Here's the drawing with two shaded views (mm, measured from the low corner). I have some questions. Round coordinates to 2 decimals unless told otherwise and drop trailing zeros. Order: outer loops, then holes, each group sorted by start corner. A loop starts at its lowest first (then second) coordinate and runs counter-clockwise, first axis right, second up. Notation, with made-up numbers: (-32.5, 65.25) -> (23.5, 65.25) arc R16 cw to (23.5, 87.25) -> close; hole circle Ø1 at (78, 86.25). An arc over 180 degrees is marked (long way). One line per question, with ' | ' between items.
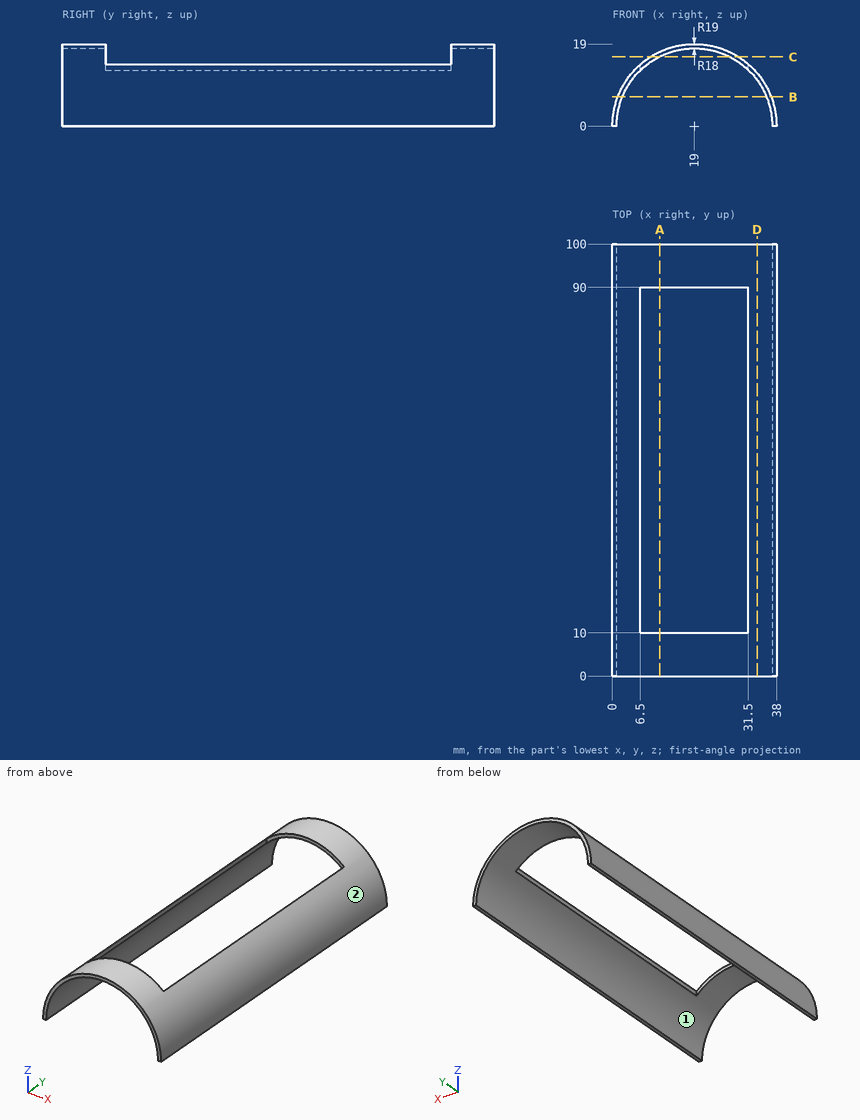
1. I want a section at C-C on z = 16. List the corners of the cut face in (x, y) for me.
From the geometry:
outline: (8.75, 0) -> (10.75, 0) -> (10.75, 10) -> (8.75, 10) -> close; (8.75, 90) -> (10.75, 90) -> (10.75, 100) -> (8.75, 100) -> close; (27.25, 0) -> (29.25, 0) -> (29.25, 10) -> (27.25, 10) -> close; (27.25, 90) -> (29.25, 90) -> (29.25, 100) -> (27.25, 100) -> close
2. I want a section at A-A on x = 11. List the corners of the cut face in (y, z) for me.
From the geometry:
outline: (0, 16.12) -> (10, 16.12) -> (10, 17.23) -> (0, 17.23) -> close; (90, 16.12) -> (100, 16.12) -> (100, 17.23) -> (90, 17.23) -> close
3. If we mould it in two halves opening along X, with no side actions, what happens to the marked faces 1 and 2? For each: pulls with the +X half, pulls with the -X half, needs draft (parallel to the pull), parting line crosses it, or undercut.
From the geometry:
face 1: undercut | face 2: parting line crosses it
4. I want a section at B-B on z = 6.75. List the corners of the cut face in (x, y) for me, and give its area (3 significant figures).
From the geometry:
outline: (1.24, 0) -> (2.31, 0) -> (2.31, 100) -> (1.24, 100) -> close; (35.69, 0) -> (36.76, 0) -> (36.76, 100) -> (35.69, 100) -> close | area: 215 mm²
5. I'm going to push flat-ended pins straight in: pin 1 (3 mm diameter, centred on x = 21.5, z = 15.5, fed in from +Y); pin 2 (1 mm diameter, centred on y = 11, z = 10.5, fed in from -X); pin 3 (1.5 mm diameter, centred on x = 4, y = 23, fed in from +Z); pin 4 (3 mm diameter, centred on x = 14.5, z = 17, fed in from -Y). Where does each tip first touch, or does it pass through?
From the geometry:
pin 1: passes through | pin 2: stops at x = 2.84 | pin 3: stops at z = 12.57 | pin 4: stops at y = 0
6. I want a section at D-D on x = 33.5. List the corners of the cut face in (y, z) for me, and give its area (3 significant figures).
From the geometry:
outline: (0, 10.67) -> (100, 10.67) -> (100, 12.28) -> (0, 12.28) -> close | area: 161 mm²
7. I need wall thicknesses on probe 1 along X at (y, z) = (9.5, 3.25); probe 2 along X at (y, z) = (50, 3.75); probe 3 along Z at (x, y) = (19.5, 5.5). Which ranges of each line are inside material? Lowest first, please.
From the geometry:
probe 1: x = 0.28 to 1.3, 36.7 to 37.72 | probe 2: x = 0.37 to 1.39, 36.61 to 37.63 | probe 3: z = 17.99 to 18.99
